Part model, mm, in its own coordinate system. Face numbers are marked on the shaded views. A direction names the side the tool comes from. Coordinates: 2 decimals unless noted, no trailing zeros. Loops run counter-clockwise (first coordinate to the right, second up) from the corner with the lowest first, then second, coordinate; pieces in that order, holes last. Notation, with made-up numbers: M 8,41 L 23,41 A16 ccw 23,57 Z; hole C -10.5,0 d10. An arc over 180 degrees is marked long. Use a Markdown table: item, result. Add a question column.
1) Pin check, flat tips, straight feed: pin 1 Ø7 at (x, z) = (0, 0) entering from -Y; pin 2 Ø3 at (y, z) = (1, 4) entering from -X; pin 3 Ø3 at (x, y) = (-1.5, -0.5) entering from -Z; pin 4 Ø2.5 at (x, z) = (0, 0) entering from +Y. Stop position of each tip, or through.
2) Band-saw the part on A-A (y = -1). List the corners of the cut face in (x, z), plus the area to 3 significant figures.
3) Wall check: probe 1 along X at (y, z) = (3.9, 0); probe 2 along Y at (x, z) = (3.75, -4.5). Give the ranges that are in metal, low to high. Write a range as from..to.
4) Tool access for the marked faces 1, 2 and 3: list every direction of +Z, -Z, +X, -X, +Y, -Y with a clear straight run to the whole face (end or side of a thin tool).
5) Pull direction X, two halves, no side cores. Call the marked faces 4, 5, 6 and 7: released by +X, released by -X, zero draft, split by the parting line, or undercut.
from build123d import *

# Parameters (mm, degrees)
CHAMFER1_SIZE      = 0.1
SKETCH2_R          = 4
SKETCH2_R_2        = 2.25
CUT_EXTRUDE1_DEPTH = 0.5


with BuildPart() as part:
    # Sketch1 → Revolve1 (revolve)
    with BuildSketch(Plane(origin=(0, 0, 0), x_dir=(0, 0, -1), z_dir=(1, 0, 0))):
        Polygon((1.5, -4.25), (1.5, 4.25), (6.5, 4.25), (6.5, 3.25), (4.75, 3.25), (4.75, -3.25), (6.5, -3.25), (6.5, -4.25), align=None)
    revolve(axis=Axis((0, 0, 0), (0, 1, 0)))

    # Chamfer1
    chamfer1_edges = [part.edges().sort_by_distance(p)[0] for p in [
        (0, -4.25, 1.5),
        (0, -4.25, 6.5),
        (0, -3.25, 6.5),
        (0, 3.25, 6.5),
        (0, 4.25, 6.5),
        (0, 4.25, 1.5),
    ]]
    chamfer(chamfer1_edges, length=CHAMFER1_SIZE)

    # Sketch2 → Cut-Extrude1 (cut)
    with BuildSketch(Plane(origin=(0, 4.25, 0), x_dir=(1, 0, 0), z_dir=(0, 1, 0))):
        Circle(SKETCH2_R)
        Circle(SKETCH2_R_2, mode=Mode.SUBTRACT)
    cut_extrude1 = extrude(amount=-CUT_EXTRUDE1_DEPTH, mode=Mode.SUBTRACT)

    # Mirror1: Cut-Extrude1 across plane
    add(cut_extrude1.mirror(Plane.ZX), mode=Mode.SUBTRACT)


solid = part.part
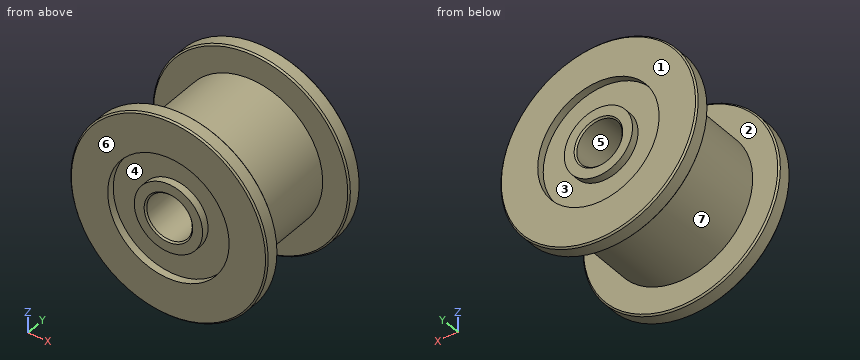
Entries:
| question | item | result |
|---|---|---|
| 1 | pin 1 | y = -4.25 |
| 1 | pin 2 | x = -4.04 |
| 1 | pin 3 | z = -4.75 |
| 1 | pin 4 | through |
| 2 | outline | C 0,0 d9.5; hole C 0,0 d3 |
| 2 | area | 63.8 mm2 |
| 3 | probe 1 | -6.5..-4, -2.25..-1.5, 1.5..2.25, 4..6.5 |
| 3 | probe 2 | -4.25..-3.25, 3.25..4.25 |
| 4 | face 1 | +Z, -Z, +X, -X, +Y |
| 4 | face 2 | none |
| 4 | face 3 | +Y |
| 5 | face 4 | undercut |
| 5 | face 5 | undercut |
| 5 | face 6 | zero draft |
| 5 | face 7 | split by the parting line |
